from build123d import *

# Parameters (mm, degrees)
F4_DEPTH  = 5
F5_W      = 65
F5_H      = 67
F7_DEPTH  = 30
F8_W      = 5
F8_H      = 20
F8_W_2    = 15
F8_H_2    = 5
F9_DEPTH  = 4
F6_W      = 3.6
F6_H      = 3.6
F10_DEPTH = 30
F11_W     = 4
F11_H     = 10
F11_W_2   = 10
F11_H_2   = 3
F12_DEPTH = 3
F13_W     = 10
F13_H     = 4
F13_W_2   = 4
F13_H_2   = 8
F14_DEPTH = 10
F3_R      = 0.889
F3_R_2    = 1.143
F3_R_3    = 2.9
F15_DEPTH = 30.001
F16_W     = 10
F16_H     = 10
F17_DEPTH = 3.5


with BuildPart() as f4:
    # F1 (on Front) → F4 (new body)
    with BuildSketch(Plane.XZ):
        Polygon((51.625, -32.5), (51.625, 37.5), (-28.375, 37.5), (-28.375, -32.5), (-28.375, -38.5), (51.625, -38.5), align=None)
    extrude(amount=F4_DEPTH)

    # F5 (on Front) → F7 (join)
    with BuildSketch(Plane.XZ):
        Polygon((45.625, 37.5), (-22.375, 37.5), (-22.375, -32.5), (45.625, -32.5), (45.625, -26.5), align=None)
        with Locations((11.625, 2.5)):
            Rectangle(F5_W, F5_H, mode=Mode.SUBTRACT)
    extrude(amount=F7_DEPTH)

    # F8 (on face) → F9 (cut)
    with BuildSketch(Plane.XZ.offset(5)):
        with Locations((-18.375, -16.5)):
            Rectangle(F8_W, F8_H)
        with Locations((1.625, -28.5)):
            Rectangle(F8_W_2, F8_H_2)
        with Locations((21.625, -28.5)):
            Rectangle(F8_W_2, F8_H_2)
        with Locations((41.625, -16.5)):
            Rectangle(F8_W, F8_H)
    extrude(amount=-F9_DEPTH, mode=Mode.SUBTRACT)

    # F6 (on Front) → F10 (join)
    with BuildSketch(Plane.XZ):
        with Locations((-20.575, 35.7)):
            Rectangle(F6_W, F6_H)
        with Locations((43.825, 35.7)):
            Rectangle(F6_W, F6_H)
        with Locations((-20.575, -30.7)):
            Rectangle(F6_W, F6_H)
        with Locations((43.825, -30.7)):
            Rectangle(F6_W, F6_H)
    extrude(amount=F10_DEPTH)

    # F11 (on face) → F12 (cut)
    with BuildSketch(Plane.XZ.offset(5)):
        with Locations((-21.875, -16.5)):
            Rectangle(F11_W, F11_H)
        with Locations((45.125, -16.5)):
            Rectangle(F11_W, F11_H)
        with Locations((21.625, -32.5)):
            Rectangle(F11_W_2, F11_H_2)
        with Locations((1.625, -32.5)):
            Rectangle(F11_W_2, F11_H_2)
    extrude(amount=F12_DEPTH, mode=Mode.SUBTRACT)

    # F13 (on face) → F14 (cut)
    with BuildSketch(Plane.XZ.offset(30)):
        with Locations((11.625, 35.5)):
            Rectangle(F13_W, F13_H)
        with Locations((-20.375, 27.5)):
            Rectangle(F13_W_2, F13_H_2)
        with Locations((-20.375, 9.5)):
            Rectangle(F13_W_2, F13_H_2)
        with Locations((43.625, 27.5)):
            Rectangle(F13_W_2, F13_H_2)
        with Locations((43.625, 9.5)):
            Rectangle(F13_W_2, F13_H_2)
    extrude(amount=-F14_DEPTH, mode=Mode.SUBTRACT)

    # F3 (on Front) → F15 (cut, through all)
    with BuildSketch(Plane.XZ):
        with Locations((-11.875, -10.5)):
            Circle(F3_R)
        with Locations((-25.875, -10.5)):
            Circle(F3_R)
        with Locations((-25.875, -22.5)):
            Circle(F3_R)
        with Locations((-11.875, -22.5)):
            Circle(F3_R)
        with Locations((-25.375, -29.5)):
            Circle(F3_R_2)
        with Locations((-25.375, 34.5)):
            Circle(F3_R_2)
        with Locations((48.625, 34.5)):
            Circle(F3_R_2)
        with Locations((35.125, -10.5)):
            Circle(F3_R)
        with Locations((35.125, -22.5)):
            Circle(F3_R)
        with Locations((49.125, -10.5)):
            Circle(F3_R)
        with Locations((49.125, -22.5)):
            Circle(F3_R)
        with Locations((48.625, -29.5)):
            Circle(F3_R_2)
        with Locations((-20.575, 35.7)):
            Circle(F3_R)
        with Locations((43.825, 35.7)):
            Circle(F3_R)
        with Locations((-20.575, -30.7)):
            Circle(F3_R)
        with Locations((-4.375, -22)):
            Circle(F3_R)
        with Locations((7.625, -22)):
            Circle(F3_R)
        with Locations((-4.375, -36)):
            Circle(F3_R)
        with Locations((7.625, -36)):
            Circle(F3_R)
        with Locations((15.625, -22)):
            Circle(F3_R)
        with Locations((27.625, -22)):
            Circle(F3_R)
        with Locations((27.625, -36)):
            Circle(F3_R)
        with Locations((15.625, -36)):
            Circle(F3_R)
        with Locations((43.825, -30.7)):
            Circle(F3_R)
        with Locations((-6.375, 27.5)):
            Circle(F3_R_3)
    extrude(amount=F15_DEPTH, mode=Mode.SUBTRACT)

    # F16 (on Front) → F17 (cut)
    with BuildSketch(Plane.XZ):
        with Locations((-6.375, 27.5)):
            Rectangle(F16_W, F16_H)
    extrude(amount=F17_DEPTH, mode=Mode.SUBTRACT)


solid = f4.part
Model file for the job. Use its own axes, mm. A direction names the side the tool comes from. Round coordinates to 2 decimals unless told otherwise and drop trailing zeros. Loops run counter-clockwise (first coordinate to the right, second up) from the corner with the lowest first, then second, coordinate; pieces in that order, holes last.
1. Band-saw the part on B-B, the plane z = -20. List the corners of the cut face in (x, y) (3 decimals), and give its area (3 significant figures).
Check values:
outline: (-28.375, -5) - (-20.875, -5) - (-20.875, -1) - (-15.875, -1) - (-15.875, -5) - (39.125, -5) - (39.125, -1) - (44.125, -1) - (44.125, -5) - (51.625, -5) - (51.625, 0) - (-28.375, 0) - close; (-22.375, -30) - (-20.875, -30) - (-20.875, -8) - (-22.375, -8) - close; (44.125, -30) - (45.625, -30) - (45.625, -8) - (44.125, -8) - close
area: 426 mm2
2. Tool access for faces 1 (the flat face through (-11.375, -2, 27)), 2 (the cylindrical face through (-25.623, -2.465, 33.384)), 3 (the flat face through (42, -3, -6.5)): list every direction of +Z, -Z, +X, -X, +Y, -Y with a clear straight run to the whole face (end or side of a thin tool).
Check values:
face 1: +Y
face 2: +Y, -Y
face 3: -Y
3. Band-saw the part on C-C, the plane z = 27.5. List the corners of the cut face in (x, y) (3 decimals).
Check values:
outline: (-28.375, -5) - (-22.375, -5) - (-22.375, -20) - (-20.875, -20) - (-20.875, -5) - (-9.275, -5) - (-9.275, -3.5) - (-11.375, -3.5) - (-11.375, 0) - (-28.375, 0) - close; (-3.475, -5) - (44.125, -5) - (44.125, -20) - (45.625, -20) - (45.625, -5) - (51.625, -5) - (51.625, 0) - (-1.375, 0) - (-1.375, -3.5) - (-3.475, -3.5) - close
4. Band-saw the part on A-A, the plane x = 20. List the corners of the cut face in (y, z), and give its area (4 significant figures).
Check values:
outline: (-30, -32.5) - (-8, -32.5) - (-8, -31) - (-30, -31) - close; (-30, 36) - (-5, 36) - (-5, -26) - (-1, -26) - (-1, -31) - (-5, -31) - (-5, -38.5) - (0, -38.5) - (0, 37.5) - (-30, 37.5) - close
area: 430.5 mm2
5. Drop flat-ended pins along their axis: P1, Ø1, axis at x = 36, y = -15.5, coming from the -Z side; P2, Ø1.7, axis at y = -17.5, z = 34.5, coming from the -X side (3 decimals); P3, Ø3, axis at x = 49.125, z = -22.5, coming from the -Y side. Give the stop position or say it passes through.
Check values:
P1: stops at z = -32.5
P2: stops at x = -22.375
P3: stops at y = -5
6. Band-saw the part on D-D, the plane y = -6.5. Count the separate pieces of the cut face and the enclosed holes in it, and give its area (3 significant figures).
Check values:
separate pieces: 4
enclosed holes: 4
area: 353 mm2
7. Wall check: probe 1 along X at (y, z) = (-1.5, -36) (3 decimals); probe 2 along X at (y, z) = (-18, -30.7) (3 decimals); probe 3 along X at (y, z) = (-1.45, 34.5) (3 decimals). Give the ranges that are in metal, low to high.
Check values:
probe 1: x = -28.375 to -5.264, -3.486 to 6.736, 8.514 to 14.736, 16.514 to 26.736, 28.514 to 51.625
probe 2: x = -22.375 to -21.464, -19.686 to -18.775, 42.025 to 42.936, 44.714 to 45.625
probe 3: x = -28.375 to -26.518, -24.232 to 47.482, 49.768 to 51.625
8. Mould opens along Z. For faces 4 (the flat face through (-6, -2, 32.5)), 5 (the flat face through (-28.375, -2, 0)), 6 (the flat face through (12, -15, 37.5)), 7 (the cylindrical face through (7.51, -2.46, -21.12)) say: +Z half, -Z half, draft (parallel to the pull), parting line (faces both ways), or undercut.
Check values:
face 4: undercut
face 5: draft
face 6: +Z half
face 7: undercut
